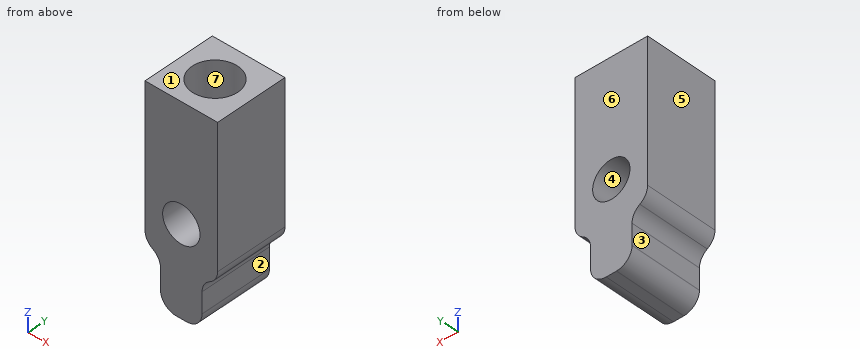
from build123d import *

# Parameters (mm, degrees)
SKETCH1_W           = 7
SKETCH1_H           = 19.5
BOSS_EXTRUDE1_DEPTH = 7
CUT_EXTRUDE1_DEPTH  = 8
CUT_EXTRUDE2_DEPTH  = 8
FILLET1_R           = 1.5
CUT_EXTRUDE3_REACH  = 9
SKETCH4_R           = 1.8
SKETCH5_R           = 2.2
CUT_EXTRUDE4_DEPTH  = 7


with BuildPart() as part:
    # Sketch1 → Boss-Extrude1 (new body)
    with BuildSketch(Plane(origin=(-3.5, 0, 0), x_dir=(0, -1, 0), z_dir=(-1, 0, 0))):
        with Locations((-5, 1.25)):
            Rectangle(SKETCH1_W, SKETCH1_H)
    extrude(amount=-BOSS_EXTRUDE1_DEPTH)

    # Sketch2 → Cut-Extrude1 (cut, through all)
    with BuildSketch(Plane(origin=(0, 8.5, 0), x_dir=(-1, 0, 0), z_dir=(0, 1, 0))):
        with BuildLine():
            Line((-3.5, -2.401923806), (-3.5, -8.5))
            Line((-3.5, -8.5), (-2.00000003, -8.5))
            Line((-2.00000003, -8.5), (-2.00000003, -5))
            ThreePointArc((-2.00000003, -5), (-2.20096192, -4.250000007), (-2.750000015, -3.700961903))
            ThreePointArc((-2.750000015, -3.700961903), (-3.29903811, -3.151923798), (-3.5, -2.401923806))
        make_face()
    extrude(amount=-CUT_EXTRUDE1_DEPTH, mode=Mode.SUBTRACT)

    # Sketch3 → Cut-Extrude2 (cut, through all)
    with BuildSketch(Plane(origin=(0, 8.5, 0), x_dir=(-1, 0, 0), z_dir=(0, 1, 0))):
        with BuildLine():
            Line((1.99999997, -5), (1.99999997, -8.5))
            Line((1.99999997, -8.5), (3.5, -8.5))
            Line((3.5, -8.5), (3.5, -2.401923771))
            ThreePointArc((3.5, -2.401923771), (3.299038101, -3.151923779), (2.749999985, -3.700961886))
            ThreePointArc((2.749999985, -3.700961886), (2.200961869, -4.249999993), (1.99999997, -5))
        make_face()
    extrude(amount=-CUT_EXTRUDE2_DEPTH, mode=Mode.SUBTRACT)

    # Fillet1
    fillet1_edges = [part.edges().sort_by_distance(p)[0] for p in [
        (2.00000003, 5, -8.5),
        (-1.99999997, 5, -8.5),
    ]]
    fillet(fillet1_edges, radius=FILLET1_R)

    # Sketch4 → Cut-Extrude3 (cut, up to next)
    with BuildSketch(Plane(origin=(0, 8.5, 0), x_dir=(1, 0, 0), z_dir=(0, 1, 0)), mode=Mode.PRIVATE) as cut_extrude3_sk1:
        Circle(SKETCH4_R)
    cut_extrude3_tool1 = extrude(cut_extrude3_sk1.sketch, amount=-CUT_EXTRUDE3_REACH, mode=Mode.PRIVATE) & part.part
    add(cut_extrude3_tool1.solids().sort_by_distance((0, 8.5, 0))[0], mode=Mode.SUBTRACT)

    # Sketch5 → Cut-Extrude4 (cut)
    with BuildSketch(Plane.XY.offset(11)):
        with Locations((0, 5)):
            Circle(SKETCH5_R)
    extrude(amount=-CUT_EXTRUDE4_DEPTH, mode=Mode.SUBTRACT)


solid = part.part
Verification items for the finished model (mm, model axes). Face numbers are marked on the shaded views. A direction names the side the tool comes from. Coordinates: 2 decimals unless noted, no trailing zeros. Order: outer loops, then holes, each group sorted by start corner. A loop starts at its lowest first (then second) coordinate and runs counter-clockwise, first axis right, second up. Notation, with made-up numbers: M 77.5,-18.5 L 122.5,-18.5 A17 ccw 122.5,-12.5 Z; hole C -12.5,80.5 d6. An arc over 180 degrees is marked long. One line per item, written item: value. Start each with the question number.
Item 1: Access from +Z, -Z, +X, -X, +Y, -Y to the whole of each face (thin tool, end or side, straight path). Record for the marked faces 1, 2 and 3.
Item 2: Sectioned sample at B-B (y = 5). Enter the section's corners in (x, z).
Item 3: Mould release check, pull along X, two halves, no side actions. Record for the marked faces 4, 5, 6 and 7: released by +X, released by -X, zero draft, split by the parting line, or undercut.
Item 4: Sectioned sample at A-A (z = 0). Enter the section's corners in (x, y), then the cut area to 3 significant figures.
Item 5: Gauge pin test, flat ends, axial feed: pin 1 (0.6 mm diameter, centred on y = 4, z = -6, fed in from +X); pin 2 (1 mm diameter, centred on y = 2.5, z = -2.5, fed in from +X); pin 3 (0.6 mm diameter, centred on y = 3.5, z = -5.5, fed in from -X); pin 4 (1.3 mm diameter, centred on x = 1, y = 6, fed in from +Z). Record the tip position at first contact, or that the pin passes through.
Item 6: Sectioned sample at D-D (z = 9). Enter the section's corners in (x, y).
Item 7: Sectioned sample at C-C (x = 0). Enter the section's corners in (y, z), then the cut area to 3 significant figures.
Item 8: Scan lines: probe 1 along Y at (x, z) = (0, 6); probe 2 along X at (y, z) = (6, 0); probe 3 along Z at (x, y) = (0, 6.25). Record each from-to range of solid material in increasing order.
Conclusion:
1. face 1: +Z, +X, -X, +Y, -Y
1. face 2: -Z, +X, +Y, -Y
1. face 3: -Z, -X, +Y, -Y
2. outline: M -3.5,-2.4 A1.5 ccw -2.75,-3.7 A1.5 cw -2,-5 L -2,-7 A1.5 ccw -0.5,-8.5 L 0.5,-8.5 A1.5 ccw 2,-7 L 2,-5 A1.5 cw 2.75,-3.7 A1.5 ccw 3.5,-2.4 L 3.5,11 L 2.2,11 L 2.2,4 L -2.2,4 L -2.2,11 L -3.5,11 Z; hole C 0,0 d3.6
3. face 4: undercut
3. face 5: released by -X
3. face 6: zero draft
3. face 7: undercut
4. outline: M -3.5,1.5 L -1.8,1.5 L -1.8,8.5 L -3.5,8.5 Z; M 1.8,1.5 L 3.5,1.5 L 3.5,8.5 L 1.8,8.5 Z
4. area: 23.8 mm^2
5. pin 1: stops at x = 2
5. pin 2: stops at x = 3.5
5. pin 3: stops at x = -2
5. pin 4: stops at z = 4
6. outline: M -3.5,1.5 L 3.5,1.5 L 3.5,8.5 L -3.5,8.5 Z; hole C 0,5 d4.4
7. outline: M 1.5,-8.5 L 8.5,-8.5 L 8.5,-1.8 L 1.5,-1.8 Z; M 1.5,1.8 L 8.5,1.8 L 8.5,11 L 7.2,11 L 7.2,4 L 2.8,4 L 2.8,11 L 1.5,11 Z
7. area: 80.5 mm^2
8. probe 1: y = 1.5 to 2.8, 7.2 to 8.5
8. probe 2: x = -3.5 to -1.8, 1.8 to 3.5
8. probe 3: z = -8.5 to -1.8, 1.8 to 4
